Part print with two shaded views. Sizes in mm from the minimum x, y, z corner. Coordinates: 2 decimals unless noted, no trailing zeros. Order: outer loops, then holes, each group sorted by start corner. A loop starts at its lowest first (then second) coordinate and runs counter-clockwise, first axis right, second up. Notation, with made-up numbers: (41.25, -27) - (56.25, -27) arc R26 cw to (56.25, 10) - close; hole circle Ø11 at (71, 85). An arc over 180 degrees is marked (long way). One line per item, written item: value.
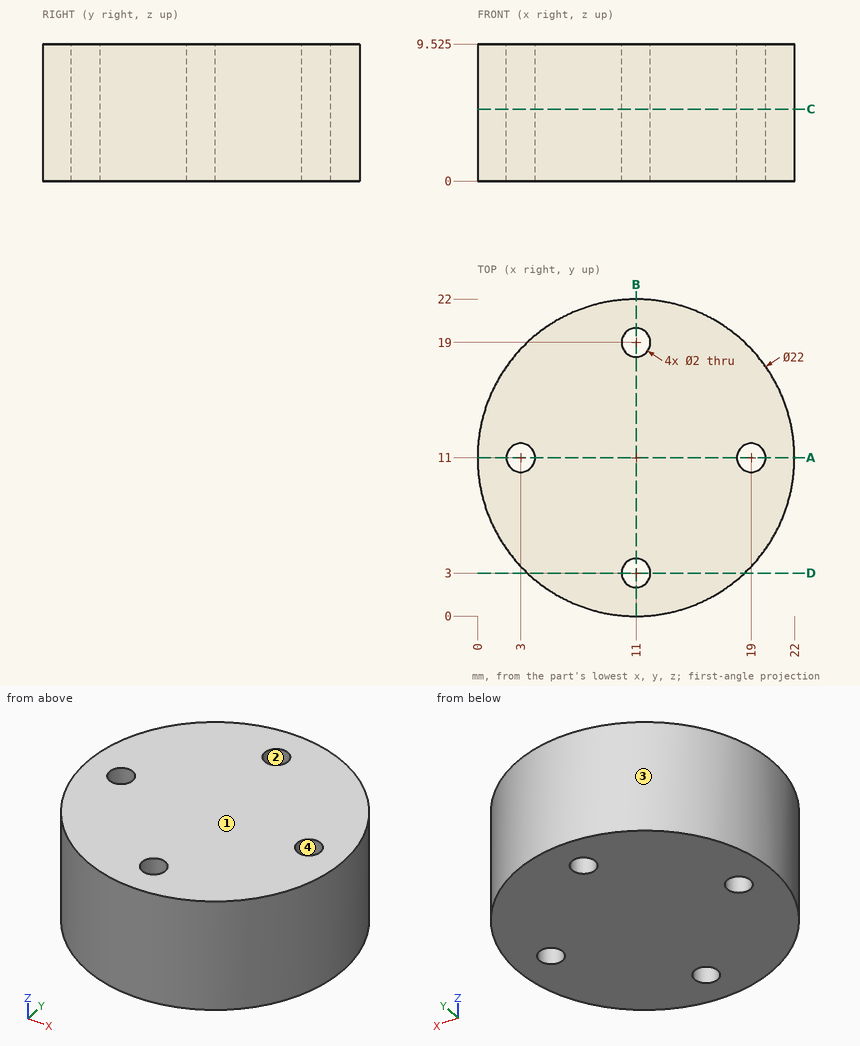
1. Two-plate mould, pull along X, no slides. Class the marked faces 1, 2, 3 and 4: pulls with the +X half, pulls with the -X half, needs draft (parallel to the pull), parting line crosses it, or undercut.
Values found:
face 1: needs draft
face 2: undercut
face 3: parting line crosses it
face 4: undercut
2. Probe line 1 along Y through (x, z) = (11, 4.75); line 2 along X through (y, z) = (10.25, 3.5); line 3 along X through (y, z) = (10.75, 5). List the from-to ranges inside material, lowest first.
Values found:
line 1: y = 0 to 2, 4 to 18, 20 to 22
line 2: x = 0.03 to 2.34, 3.66 to 18.34, 19.66 to 21.97
line 3: x = 0 to 2.03, 3.97 to 18.03, 19.97 to 22
3. Band-saw the part on A-A, the plane y = 11. Give the cut face in (x, z) (3 decimals).
Values found:
outline: (0, 0) - (2, 0) - (2, 9.525) - (0, 9.525) - close; (4, 0) - (18, 0) - (18, 9.525) - (4, 9.525) - close; (20, 0) - (22, 0) - (22, 9.525) - (20, 9.525) - close
4. Band-saw the part on C-C, the plane z = 5. Give the cut face in (x, y), and give its area (3 significant figures).
Values found:
outline: circle Ø22 at (11, 11); hole circle Ø2 at (3, 11); hole circle Ø2 at (11, 3); hole circle Ø2 at (11, 19); hole circle Ø2 at (19, 11)
area: 368 mm2
5. Band-saw the part on D-D, the plane y = 3. Give the cut face in (x, z) (3 decimals).
Values found:
outline: (3.45, 0) - (10, 0) - (10, 9.525) - (3.45, 9.525) - close; (12, 0) - (18.55, 0) - (18.55, 9.525) - (12, 9.525) - close
6. Flat gauge pins, fed straight in: P1, Ø2, axis at y = 16, z = 3.5, coming from the +X side; P2, Ø4, axis at x = 14.5, z = 8.5, coming from the -Y side; P3, Ø1, axis at y = 10, z = 2.5, coming from the +X side. Where does each tip first touch, or does it go through?
Values found:
P1: stops at x = 21.25
P2: stops at y = 0.1
P3: stops at x = 21.99
